Answer from the drawing. Dimensions are ordinates in mm from the lowest x, y and z of the part. Coordinates: 2 decimals unless noted, no trailing zeros. Loops run counter-clockwise (first coordinate to the right, second up) from the corner with the lowest first, then second, coordinate; pieces in that order, holes last. Notation, with made-up numbers: M -17.75,-2 L -10.75,-2 A26 cw -10.75,32 Z; hole C 18.5,60.5 d2. An arc over 180 degrees is marked long. Put each result on its own line as item: value.
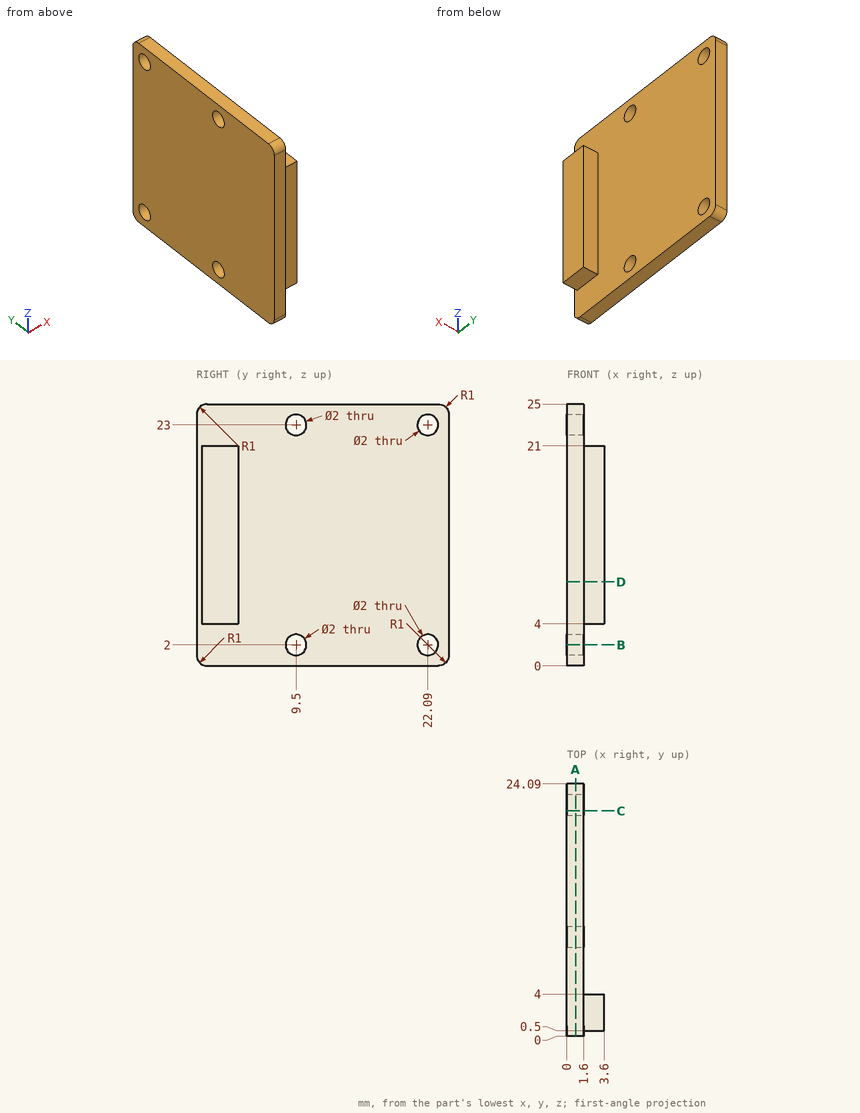
1) Straight lines are drawn through the part: line 1 (Y direction, x = 0.3, z = 23); line 2 (X direction, y = 16, z = 22); line 3 (Y direction, x = 2.2, z = 5.75). For each, find the intervals that lie inside material, in ascending order. Write a range as [from, to].
Answer list:
line 1: y = [0, 8.5], [10.5, 21.09], [23.09, 24.09]
line 2: x = [0, 1.6]
line 3: y = [0.5, 4]
2) Find section A-A, the plane x = 0.85. Write down the section's boundary in (y, z).
Answer list:
outline: M 0,1 A1 ccw 1,0 L 23.09,0 A1 ccw 24.09,1 L 24.09,24 A1 ccw 23.09,25 L 1,25 A1 ccw 0,24 Z; hole C 9.5,2 d2; hole C 9.5,23 d2; hole C 22.09,2 d2; hole C 22.09,23 d2
3) Find section C-C, the plane y = 21.5. Write down the section's boundary in (x, z).
Answer list:
outline: M 0,0 L 1.6,0 L 1.6,1.19 L 0,1.19 Z; M 0,2.81 L 1.6,2.81 L 1.6,22.19 L 0,22.19 Z; M 0,23.81 L 1.6,23.81 L 1.6,25 L 0,25 Z
4) Find section D-D, the plane z = 8. Write down the section's boundary in (x, y).
Answer list:
outline: M 0,0 L 1.6,0 L 1.6,0.5 L 3.6,0.5 L 3.6,4 L 1.6,4 L 1.6,24.09 L 0,24.09 Z
5) Given pin 1 Ø0.6 at (x, y) = (2.5, 3) entering from +Z; pin 2 Ø7 at (y, z) = (12, 9.5) entering from +X; pin 3 Ø1.6 at (x, y) = (3, 2) entering from -Z, each flat-ended and moving along its own axis, determine where each tip first touches the part or whether it passes through.
Answer list:
pin 1: stops at z = 21
pin 2: stops at x = 1.6
pin 3: stops at z = 4
6) Find section B-B, the plane z = 2. Write down the section's boundary in (x, y).
Answer list:
outline: M 0,0 L 1.6,0 L 1.6,8.5 L 0,8.5 Z; M 0,10.5 L 1.6,10.5 L 1.6,21.09 L 0,21.09 Z; M 0,23.09 L 1.6,23.09 L 1.6,24.09 L 0,24.09 Z
